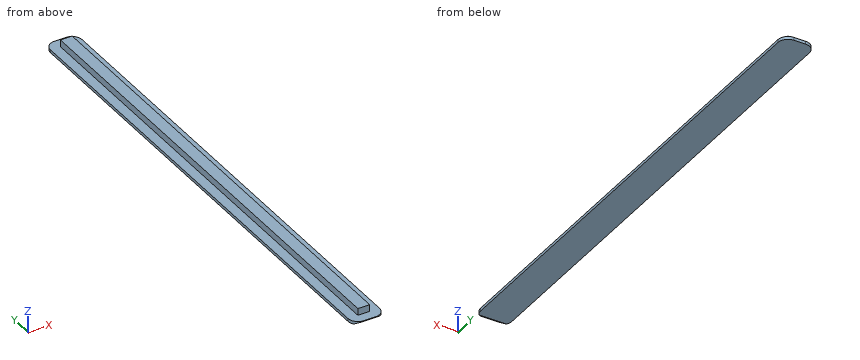
from build123d import *

# Parameters (mm, degrees)
F0_W        = 6.4
F0_H        = 104
F0_W_2      = 2.4
F0_H_2      = 100
F1_DEPTH    = 0.6
F2_DEPTH    = 2
F3_R        = 2
F4_T1_DEPTH = 6.5393372074


# Not quite as in the source:
# - a fillet or chamfer that OpenCascade refuses, or shapes differently, is made with other operations: its cross-section is extruded or revolved along the edge and cut away or added


with BuildPart() as f1:
    # F0 (on Top) → F1 (new body)
    with BuildSketch(Plane.XY):
        Rectangle(F0_W, F0_H)
        Rectangle(F0_W_2, F0_H_2, mode=Mode.SUBTRACT)
    extrude(amount=F1_DEPTH)

    # F0 (on Top) → F2 (join)
    with BuildSketch(Plane.XY):
        Rectangle(F0_W_2, F0_H_2)
    extrude(amount=F2_DEPTH)

    # F3
    f3_edges = [f1.edges().sort_by_distance(p)[0] for p in [
        (-3.2, -52, 0.3),
        (-3.2, 52, 0.3),
        (3.2, 52, 0.3),
        (3.2, -52, 0.3),
    ]]
    fillet(f3_edges, radius=F3_R)

    # F4: chamfer of 0.8 x 0.4618802154 on 1 edges, made by hand

    # F4_s2 → F4_t1 (cut)
    with BuildSketch(Plane.YZ.offset(-3.2696686037)):
        Polygon((-51.2, 0), (-52, 0.4618802154), (-52, 0), align=None)
    extrude(amount=F4_T1_DEPTH, mode=Mode.SUBTRACT)


solid = f1.part
Could you check a few things on this model? Use its own coordinates, in mm. Round coordinates to 2 decimals unless told otherwise and drop trailing zeros. Order: outer loops, then holes, each group sorted by start corner. A loop starts at its lowest first (then second) coordinate and runs counter-clockwise, first axis right, second up.
(1) Imagine slicing it at A-A (y = 18). Write out the boundary of the cut face in (x, z).
Response values:
outline: (-3.2, 0) - (3.2, 0) - (3.2, 0.6) - (1.2, 0.6) - (1.2, 2) - (-1.2, 2) - (-1.2, 0.6) - (-3.2, 0.6) - close
(2) Please list where these lines run through material, in increasing order: line 1 along Z through (x, y) = (-2, 5); line 2 along Y through (x, z) = (-0.5, 1.25); line 3 along X through (y, z) = (39, 1.65).
Response values:
line 1: z = 0 to 0.6
line 2: y = -50 to 50
line 3: x = -1.2 to 1.2
(3) Imagine slicing it at B-B (z = 1.2). Write out the boundary of the cut face in (x, y).
Response values:
outline: (-1.2, -50) - (1.2, -50) - (1.2, 50) - (-1.2, 50) - close
(4) I'm going to push flat-ended pins straight in: pin 1 (1.1 mm diameter, centred on y = 8, z = 1.5, fed in from +X); pin 2 (1.1 mm diameter, centred on x = -0.5, z = 1, fed in from -Y); pin 3 (0.7 mm diameter, centred on x = 0.5, z = 1.5, fed in from +Y). Where does each tip first touch, or does it pass through?
Response values:
pin 1: stops at x = 1.2
pin 2: stops at y = -52
pin 3: stops at y = 50
